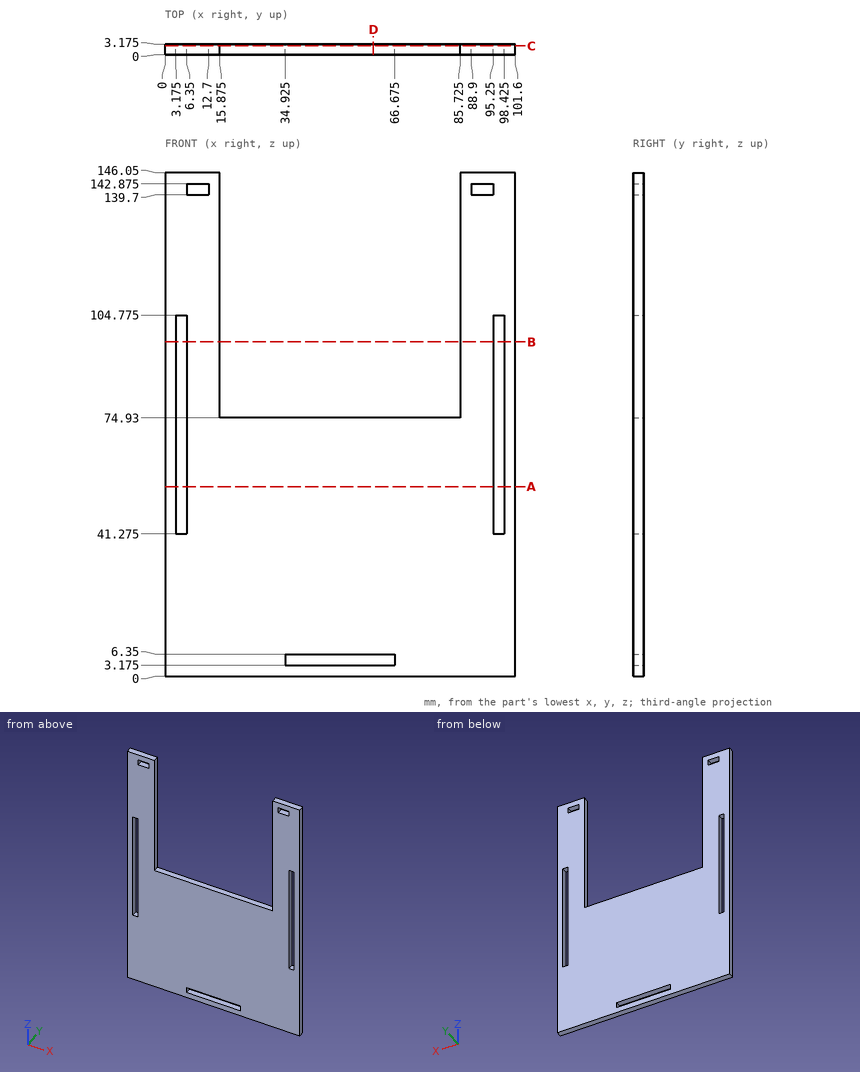
Geometry check sheet. Reference: drawing and pictorial views, mm from the part's lowest x, y, z. Give positions to 0.01 mm unless a question says otherwise; leave off trailing zeros. Order: outer loops, then holes, each group sorted by start corner. A loop starts at its lowest first (then second) coordinate and runs counter-clockwise, first axis right, second up. Notation, with made-up numbers: M -17.5,52.25 L 39.5,52.25 A24 cw 39.5,72.25 Z; hole C 76.25,33.5 d11. An arc over 180 degrees is marked long. Answer in a Markdown table with one row per item. Add a question column.
Q1. Thickness scan on L1, parallel to X at y = 1.4, z = 53.5 (3 decimals); L2, parallel to X at y = 2.3, z = 108 (3 decimals); L3, parallel to Z at x = 63, y = 2.85 (3 decimals). Record the ranges inside material, lowest first.
Q2. Sectioned sample at A-A, the plane z = 55. Record the boundary of the cut face in (x, y) (3 decimals), and give its area (3 significant figures).
Q3. Gauge pin test, flat end, axial feed: pin 1 Ø1 at (x, y) = (47.5, 1) entering from +Z. Record the tip position at first contact, or that the pin passes through.
Q4. Sectioned sample at B-B, the plane z = 97. Record the boundary of the cut face in (x, y) (3 decimals).
Q5. Sectioned sample at C-C, the plane y = 2.6. Record the boundary of the cut face in (x, z) (3 decimals).
Q6. Sectioned sample at D-D, the plane x = 60.5. Record the boundary of the cut face in (y, z) (3 decimals).
Verdict:
| question | item | result |
|---|---|---|
| 1 | L1 | 0 to 3.175, 6.35 to 95.25, 98.425 to 101.6 |
| 1 | L2 | 0 to 15.875, 85.725 to 101.6 |
| 1 | L3 | 0 to 3.175, 6.35 to 74.93 |
| 2 | outline | M 0,0 L 3.175,0 L 3.175,3.175 L 0,3.175 Z; M 6.35,0 L 95.25,0 L 95.25,3.175 L 6.35,3.175 Z; M 98.425,0 L 101.6,0 L 101.6,3.175 L 98.425,3.175 Z |
| 2 | area | 302 mm² |
| 3 | pin 1 | z = 74.93 |
| 4 | outline | M 0,0 L 3.175,0 L 3.175,3.175 L 0,3.175 Z; M 6.35,0 L 15.875,0 L 15.875,3.175 L 6.35,3.175 Z; M 85.725,0 L 95.25,0 L 95.25,3.175 L 85.725,3.175 Z; M 98.425,0 L 101.6,0 L 101.6,3.175 L 98.425,3.175 Z |
| 5 | outline | M 0,0 L 101.6,0 L 101.6,146.05 L 85.725,146.05 L 85.725,74.93 L 15.875,74.93 L 15.875,146.05 L 0,146.05 Z; hole M 3.175,41.275 L 6.35,41.275 L 6.35,104.775 L 3.175,104.775 Z; hole M 6.35,139.7 L 12.7,139.7 L 12.7,142.875 L 6.35,142.875 Z; hole M 34.925,3.175 L 66.675,3.175 L 66.675,6.35 L 34.925,6.35 Z; hole M 88.9,139.7 L 95.25,139.7 L 95.25,142.875 L 88.9,142.875 Z; hole M 95.25,41.275 L 98.425,41.275 L 98.425,104.775 L 95.25,104.775 Z |
| 6 | outline | M 0,0 L 3.175,0 L 3.175,3.175 L 0,3.175 Z; M 0,6.35 L 3.175,6.35 L 3.175,74.93 L 0,74.93 Z |
